Geometry check sheet. Reference: the model listing, model coordinates, mm. A direction names the side the tool comes from. Give positions to 0.01 mm unless a question says otherwise; leave off trailing zeros. Write each loop counter-clockwise with the first axis right and the second up, starting at its lowest first coordinate (ties: lowest second). Pieces come first, ordered by that corner, then holes. Notation, with made-up numbers: (49.5, 66.25) -> (99.5, 66.25) arc R9 cw to (99.5, 73.25) -> close; hole circle Ø1 at (3, -32). An arc over 180 degrees is marked (long way). Use a Markdown table: item, result. Add a question column.
from build123d import *

# Parameters (mm, degrees)
F1_DEPTH = 25.4
F3_DEPTH = 12.7
F5_DEPTH = 12.7
F6_W     = 3.653213
F6_H     = 3.617645
F6_W_2   = 4.803298
F6_H_2   = 4.835383
F7_DEPTH = 12.7


with BuildPart() as f1:
    # F0 (on Front) → F1 (new body)
    with BuildSketch(Plane.XZ):
        with BuildLine():
            ThreePointArc((5.963441, 35.366944), (-27.388586, -23.157045), (35.866187, 0))
            ThreePointArc((35.866187, 0), (28.988599, 21.119765), (10.993484, 34.13981))
            ThreePointArc((10.993484, 34.13981), (8.500635, 34.844261), (5.963441, 35.366944))
        make_face()
        with BuildLine():
            ThreePointArc((5.963441, 35.366944), (8.500635, 34.844261), (10.993484, 34.13981))
            Line((10.993484, 34.13981), (12.279672, 36.955047))
            Line((12.279672, 36.955047), (13.718993, 39.114028))
            Line((13.718993, 39.114028), (15.69806, 41.992676))
            Line((15.69806, 41.992676), (17.137382, 43.97174))
            Line((17.137382, 43.97174), (18.651877, 44.50046))
            Line((18.651877, 44.50046), (16.949486, 48.106024))
            Line((16.949486, 48.106024), (13.131301, 46.303242))
            Line((13.131301, 46.303242), (9.940774, 40.91318))
            Line((9.940774, 40.91318), (5.963441, 35.366944))
        make_face()
    extrude(amount=F1_DEPTH)

    # F2 (on face) → F3 (cut)
    with BuildSketch(Plane.XZ.offset(25.4)):
        Polygon((-10.563217, 12.250198), (-16.440853, 22.498386), (-23.222743, 12.250198), align=None)
        Polygon((20.030638, 12.250198), (12.94733, 22.498386), (8.72749, 12.250198), align=None)
    extrude(amount=-F3_DEPTH, mode=Mode.SUBTRACT)

    # F4 (on face) → F5 (cut)
    with BuildSketch(Plane.XZ.offset(25.4)):
        Polygon((21.387015, -2.669957), (-20.359278, -2.669957), (0, -28.591841), align=None)
    extrude(amount=-F5_DEPTH, mode=Mode.SUBTRACT)

    # F6 (on face) → F7 (join)
    with BuildSketch(Plane.XZ.offset(12.7)):
        with Locations((-12.206394, -4.478779)):
            Rectangle(F6_W, F6_H)
        with Locations((5.755238, -5.087648)):
            Rectangle(F6_W_2, F6_H_2)
    extrude(amount=F7_DEPTH)


solid = f1.part
1) Sectioned sample at C-C, the plane y = -9.5. Enter the section's corners in (x, z), and give its area (3 significant figures).
2) Sectioned sample at B-B, the plane x = -22. Enter the section's corners in (y, z), and give its area (3 significant figures).
3) Tool access check on faces 1 (the face through (14.695, -12.522, 40.533)), 2 (the face through (-10.32, -19.14, -15.45)), 3 (the face through (-1, -25.4, 7)). Record the directions out of +Z, -Z, +X, -X, +Y, -Y that give a thin tool (end or side, any length) a straight path to the whole face; none if there is none.
4) Material ranges on probe 1 along Z at (x, y) = (15, -22.5); probe 2 along Z at (x, y) = (-18, -24); probe 3 along Y at (x, z) = (13, 21), recorded low to high. Write a range as [from, to].
5) Sectioned sample at A-A, the plane y = -14.5. Enter the section's corners in (x, z), and give its area (3 significant figures).
6) Sectioned sample at D-D, the plane z = -21. Enter the section's corners in (x, y), and give its area (3 significant figures).
7) Draft check along X on faces 4 (the face through (17.81, -12.52, 46.28)), 5 (the face through (11.56, -12.52, 43.65)), 6 (the face through (15, -19, -2.67)). Enter one of: +X half, -X half, draft (parallel to the pull), parting line (faces both ways), or undercut.
8) Gauge pin test, flat ends, axial feed: P1, Ø2, axis at y = -11.5, z = 10.5, coming from the +X side; P2, Ø4, axis at x = -0.5, y = -18, coming from the -Z side; P3, Ø4, axis at x = 5, y = -16.5, coming from the -Z side; P4, Ø13, axis at x = 9, z = -12, coming from the -Y side. Record the tip position at first contact, or that the pin passes through.
Check values:
| question | item | result |
|---|---|---|
| 1 | outline | (5.96, 35.37) arc R35.87 ccw (long way) to (10.99, 34.14) -> (12.28, 36.96) -> (13.72, 39.11) -> (15.7, 41.99) -> (17.14, 43.97) -> (18.65, 44.5) -> (16.95, 48.11) -> (13.13, 46.3) -> (9.94, 40.91) -> close |
| 1 | area | 4,110 mm² |
| 2 | outline | (-25.4, -28.33) -> (0, -28.33) -> (0, 28.33) -> (-25.4, 28.33) -> (-25.4, 14.1) -> (-12.7, 14.1) -> (-12.7, 12.25) -> (-25.4, 12.25) -> close |
| 2 | area | 1,420 mm² |
| 3 | face 1 | +X, +Y, -Y |
| 3 | face 2 | -Y |
| 3 | face 3 | +Z, -Z, +X, -X, -Y |
| 4 | probe 1 | [-32.58, -10.41], [-2.67, 12.25], [19.53, 32.58], [40.98, 47.19] |
| 4 | probe 2 | [-31.02, -5.67], [-2.67, 12.25], [20.14, 31.02] |
| 4 | probe 3 | [-12.7, 0] |
| 5 | outline | (5.96, 35.37) arc R35.87 ccw (long way) to (10.99, 34.14) -> (12.28, 36.96) -> (13.72, 39.11) -> (15.7, 41.99) -> (17.14, 43.97) -> (18.65, 44.5) -> (16.95, 48.11) -> (13.13, 46.3) -> (9.94, 40.91) -> close; hole (-23.22, 12.25) -> (-10.56, 12.25) -> (-16.44, 22.5) -> close; hole (-20.36, -2.67) -> (0, -28.59) -> (21.39, -2.67) -> (8.16, -2.67) -> (8.16, -7.51) -> (3.35, -7.51) -> (3.35, -2.67) -> (-10.38, -2.67) -> (-10.38, -6.29) -> (-14.03, -6.29) -> (-14.03, -2.67) -> close; hole (8.73, 12.25) -> (20.03, 12.25) -> (12.95, 22.5) -> close |
| 5 | area | 3,480 mm² |
| 6 | outline | (-29.08, -25.4) -> (-5.96, -25.4) -> (-5.96, -12.7) -> (6.26, -12.7) -> (6.26, -25.4) -> (29.08, -25.4) -> (29.08, 0) -> (-29.08, 0) -> close |
| 6 | area | 1,320 mm² |
| 7 | face 4 | +X half |
| 7 | face 5 | -X half |
| 7 | face 6 | undercut |
| 8 | P1 | x = 34.59 |
| 8 | P2 | z = -35.87 |
| 8 | P3 | z = -35.74 |
| 8 | P4 | y = -25.4 |
